The model under review builds one solid part; all positions refer to its coordinate system, in mm. A direction names the side the tool comes from. Round coordinates to 2 decimals unless told otherwise and drop trailing zeros. Write each loop counter-clockwise with the first axis right and the second up, starting at its lowest first coordinate (ties: lowest second). Pieces come first, ordered by that corner, then holes.
Item 1: Add section A-A (x = 0). Give the boundary of the cut face in (y, z) (3 decimals).
Item 2: Add section D-D (x = 24). Give the boundary of the cut face in (y, z) (3 decimals), plus the area to 3 significant figures.
Item 3: Draft analysis for pull direction X (two halves, no side actions). For faces 3 (the face through (1, 2, 67.945)), 4 (the face through (-39.011, -3.065, 34.448)), 5 (the face through (-45.37, -1.026, 33.497)), state which applies: +X half, -X half, draft (parallel to the pull), parting line (faces both ways), or undercut.
Item 4: Add section C-C (z = 8.5). Give the boundary of the cut face in (x, y) (3 decimals), plus the area to 3 significant figures.
Item 5: Add section B-B (y = -1). Give the boundary of the cut face in (x, z) (3 decimals), plus the area to 3 significant figures.
Item 6: Clearance check with flat-ended pins moving along their axes: pin 1 Ø1 at (y, z) = (-1.5, 26.5) entering from +X; pin 2 Ø5 at (y, z) = (1, 57) entering from +X. State where each tip first meets the part, or that it passes through.
Item 7: Machinability: for faces 1 (the face through (31.95, 0.97, 34.45)), 2 (the face through (-49, -6.35, 33)), which of the approach directions +Z, -Z, +X, -X, +Y, -Y give a long, thin tool a straight path to every point of the face, cutting with its end or side? Answer none if there is none.
Item 8: To check wall thickness, follow L1, parallel to Z at x = 0, y = 5.25 (3 decimals); L2, parallel to Y at x = -28, z = 49. State the ranges of each line that lie inside material, in increasing order.
```python
from build123d import *

# Parameters (mm, degrees)
BOSS_EXTRUDE1_DEPTH = 67.945
FILLET1_R           = 12.7
CUT_EXTRUDE1_REACH  = 89.007
CUT_EXTRUDE2_REACH  = 89.699
SKETCH5_R           = 7.62


with BuildPart() as part:
    # Sketch1 → Boss-Extrude1 (new body)
    with BuildSketch(Plane.XY):
        Polygon((-53.975, -6.35), (-33.449406604, 6.35), (33.449406604, 6.35), (53.975, -6.35), align=None)
    extrude(amount=BOSS_EXTRUDE1_DEPTH)

    # Fillet1
    fillet1_edges = [part.edges().sort_by_distance(p)[0] for p in [
        (-33.449406604, 6.35, 33.9725),
        (33.449406604, 6.35, 33.9725),
    ]]
    fillet(fillet1_edges, radius=FILLET1_R)

    # Sketch3 → Cut-Extrude1 (cut, up to next)
    with BuildSketch(Plane.XY.offset(67.945), mode=Mode.PRIVATE) as cut_extrude1_sk1:
        with BuildLine():
            Line((-51.302080212, -10.669942107), (51.302080212, -10.669942107))
            Line((51.302080212, -10.669942107), (33.847478799, 0.12991316))
            ThreePointArc((33.847478799, 0.12991316), (31.922261025, 0.979438528), (29.838099116, 1.27))
            Line((29.838099116, 1.27), (-29.838099116, 1.27))
            ThreePointArc((-29.838099116, 1.27), (-31.922261025, 0.979438528), (-33.847478799, 0.12991316))
            Line((-33.847478799, 0.12991316), (-51.302080212, -10.669942107))
        make_face()
    cut_extrude1_tool1 = extrude(cut_extrude1_sk1.sketch, amount=-CUT_EXTRUDE1_REACH, mode=Mode.PRIVATE) & part.part
    add(cut_extrude1_tool1.solids().sort_by_distance((0, -5.166229, 67.945))[0], mode=Mode.SUBTRACT)

    # Sketch5 → Cut-Extrude2 (cut, up to next)
    with BuildSketch(Plane(origin=(0, 6.35, 0), x_dir=(1, 0, 0), z_dir=(0, 1, 0)), mode=Mode.PRIVATE) as cut_extrude2_sk1:
        with Locations(Location((0, -42.545, 0), (0, 0, 180))):
            Circle(SKETCH5_R)
    cut_extrude2_tool1 = extrude(cut_extrude2_sk1.sketch, amount=-CUT_EXTRUDE2_REACH, mode=Mode.PRIVATE) & part.part
    add(cut_extrude2_tool1.solids().sort_by_distance((0, 6.35, 42.545))[0], mode=Mode.SUBTRACT)


solid = part.part
```
Numbers:
1. outline: (1.27, 0) - (6.35, 0) - (6.35, 34.925) - (1.27, 34.925) - close; (1.27, 50.165) - (6.35, 50.165) - (6.35, 67.945) - (1.27, 67.945) - close
2. outline: (1.27, 0) - (6.35, 0) - (6.35, 67.945) - (1.27, 67.945) - close
2. area: 345 mm2
3. face 3: draft
3. face 4: undercut
3. face 5: -X half
4. outline: (-53.975, -6.35) - (-44.32, -6.35) - (-33.847, 0.13) arc R7.62 cw to (-29.838, 1.27) - (29.838, 1.27) arc R7.62 cw to (33.847, 0.13) - (44.32, -6.35) - (53.975, -6.35) - (36.52, 4.45) arc R12.7 ccw to (29.838, 6.35) - (-29.838, 6.35) arc R12.7 ccw to (-36.52, 4.45) - close
4. area: 527 mm2
5. outline: (-45.328, 0) - (-35.674, 0) - (-35.674, 67.945) - (-45.328, 67.945) - close; (35.674, 0) - (45.328, 0) - (45.328, 67.945) - (35.674, 67.945) - close
5. area: 1,310 mm2
6. pin 1: stops at x = 46.94
6. pin 2: stops at x = 46.14
7. face 1: +Z, -Z, -Y
7. face 2: +Z, -Z, +X, -X, -Y
8. L1: z = 0 to 34.925, 50.165 to 67.945
8. L2: y = 1.27 to 6.35
